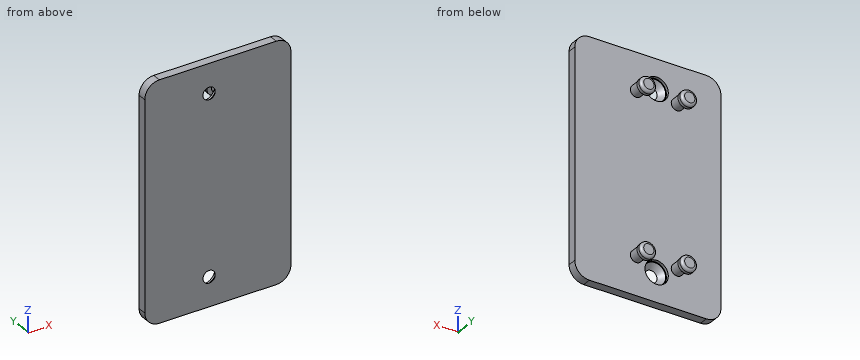
Autodesk Inventor part; units mm, degrees
ref_plane "YZ Plane" through (0, 0, 0) normal (1, 0, 0) x (0, 1, 0)
ref_plane "XZ Plane" through (0, 0, 0) normal (0, 1, 0) x (-1, 0, 0)
ref_plane "XY Plane" through (0, 0, 0) normal (0, 0, 1) x (1, 0, 0)
sketch "Esboço1" plane through (0, 0, 0) normal (0, 1, 0) x (-1, 0, 0)
  line L0 (-20, 37.5) -> (20, 37.5)
  line L1 (22, 35.5) -> (22, -35.5)
  line L2 (20, -37.5) -> (-20, -37.5)
  line L3 (-22, -35.5) -> (-22, 35.5)
  line L4 (-22, 37.5) -> (22, -37.5) construction
  line L5 (22, 37.5) -> (-22, -37.5) construction
  arc A0 (22, 35.5) -> (20, 37.5) centre (20, 35.5) ccw
  arc A1 (-20, 37.5) -> (-22, 35.5) centre (-20, 35.5) ccw
  arc A2 (-22, -35.5) -> (-20, -37.5) centre (-20, -35.5) ccw
  arc A3 (20, -37.5) -> (22, -35.5) centre (20, -35.5) ccw
  line L6 (-20, 40.5) -> (20, 40.5)
  line L7 (25, 35.5) -> (25, -35.5)
  line L8 (20, -40.5) -> (-20, -40.5)
  line L9 (-25, -35.5) -> (-25, 35.5)
  line L10 (-25, 40.5) -> (25, -40.5) construction
  line L11 (25, 40.5) -> (-25, -40.5) construction
  arc A4 (25, 35.5) -> (20, 40.5) centre (20, 35.5) ccw
  arc A5 (20, -40.5) -> (25, -35.5) centre (20, -35.5) ccw
  arc A6 (-25, -35.5) -> (-20, -40.5) centre (-20, -35.5) ccw
  arc A7 (-20, 40.5) -> (-25, 35.5) centre (-20, 35.5) ccw
  point P0 (0, 0)
  dimension "d0" = 75
  dimension "d1" = 44
  dimension "d2" = 2
  dimension "d3" = 3
  dimension "d4" = 3
  dimension "d5" = 5
extrude "Extrusão1" add sketch "Esboço1" along normal blind 3 contours L0 A0 L1 A3 L2 A2 L3 A1 | L6 A4 L7 A5 L8 A6 L9 A7
sketch "Esboço2" plane through (0, 3, 0) normal (0, 1, 0) x (1, 0, 0)
  circle A0 centre (-10, -27.5) radius 2
  circle A1 centre (-10, 27.5) radius 2
  circle A2 centre (4, -27.5) radius 2
  circle A3 centre (4, 27.5) radius 2
  line L0 (-20, -40.5) -> (20, -40.5)
  line L1 (20, 40.5) -> (-20, 40.5)
  point P0 (0, 0)
  dimension "d8" = 4
  dimension "d9" = 13
  dimension "d10" = 4
  dimension "d11" = 10
  dimension "d12" = 13
extrude "Extrusão2" add sketch "Esboço2" along normal blind 3.5
sketch "Esboço3" plane through (-10, 6.5, 27.5) normal (0, 1, 0) x (1, 0, 0)
  circle A0 centre (0, 0) radius 2
  circle A1 centre (14, 0) radius 2
  circle A2 centre (14, 55) radius 2
  circle A3 centre (0, 55) radius 2
  circle A4 centre (-0.75, 0) radius 2.75
  circle A5 centre (0, 0) radius 2
  circle A6 centre (13.25, 0) radius 2.75
  circle A7 centre (13.25, 55) radius 2.75
  circle A8 centre (-0.75, 55) radius 2.75
  circle A9 centre (0, 55) radius 2
  circle A10 centre (14, 55) radius 2
  point P0 (10, 27.5)
  dimension "d15" = 5.5
extrude "Extrusão3" add sketch "Esboço3" along normal blind 2 contours A0 | A4 | A1 | A6 | A2 | A7 | A3 | A8
fillet "Arredondamento1" radius 1 4 edges at (-13.5, 8.5, -27.5) (0.5, 8.5, -27.5) (-13.5, 8.5, 27.5) (0.5, 8.5, 27.5)
sketch "Esboço4" plane through (0, 3, 0) normal (0, 1, 0) x (1, 0, 0)
  circle A0 centre (-3, -30.5) radius 2.1
  circle A1 centre (-3, 30.5) radius 2.1
  line L0 (-20, -40.5) -> (20, -40.5)
  line L1 (20, 40.5) -> (-20, 40.5)
  line L2 (-25, 35.5) -> (-25, -35.5)
  circle A2 centre (-3, -30.5) radius 4
  circle A3 centre (-3, 30.5) radius 4
  point P0 (0, 0)
  dimension "d19" = 4.2
  dimension "d20" = 10
  dimension "d21" = 10
  dimension "d22" = 22
  dimension "d25" = 8
extrude "Extrusão4" cut sketch "Esboço4" against normal blind 10 contours A0 | A1
extrude "Extrusão5" cut sketch "Esboço4" against normal blind 1
sketch "Esboço5" plane through (-3, 2, 30.5) normal (0, 1, 0) x (1, 0, 0)
  circle A0 centre (0, 0) radius 3.75
  circle A1 centre (0, 0) radius 2.1
  circle A2 centre (0, 61) radius 4
  circle A3 centre (0, 61) radius 3.75
  point P0 (3, 30.5)
  dimension "d28" = 7.5
  dimension "d29" = 7.5
chamfer "Chanfro1" distance 2 distance2 1.65 1 edges at (-5.1, 2, 30.5) measured on face at (-0.9068, 0.6667, 30.669)
chamfer "Chanfro2" distance 2 distance2 1.65 1 edges at (-5.1, 2, -30.5) measured on face at (-0.9068, 0.6667, -30.331)
properties part number "SuportForWall"
Input: part model. Units: mm. Frame: model coordinates. Give positions to 0.01 mm unless a question says otherwise; leave off trailing zeros. Loops run counter-clockwise (first coordinate to the right, second up) from the corner with the lowest first, then second, coordinate; pieces in that order, holes last. Notation, with made-up numbers: (46, -25.75) -> (94, -25.75) arc R23 cw to (94, -1.75) -> close; hole circle Ø4 at (21, -18). An arc over 180 degrees is marked (long way). Use a Markdown table: item, result.
Q1. Section query C-C, the plane x = -15. Return the cut outline in (y, z), plus the area to 3 significant figures.
Entries:
| item | result |
|---|---|
| outline | (0, -40.5) -> (3, -40.5) -> (3, 40.5) -> (0, 40.5) -> close |
| area | 243 mm² |
Q2. Ray query, probe 1 along Z at (x, y) = (-3, 2.3); probe 2 along Z at (x, y) = (-3, 0.05); probe 3 along X at (y, z) = (2.75, -32). Return the intervals inside material, ascending. Write a range as from..to.
Entries:
| item | result |
|---|---|
| probe 1 | z = -40.5..-34.5, -26.5..26.5, 34.5..40.5 |
| probe 2 | z = -40.5..-32.64, -28.36..28.36, 32.64..40.5 |
| probe 3 | x = -25..-6.71, 0.71..25 |
Q3. Section query A-A, the plane y = 4.75. Return the cut outline in (x, z), plus the area to 3 significant figures.
Entries:
| item | result |
|---|---|
| outline | circle Ø4 at (-10, -27.5); circle Ø4 at (-10, 27.5); circle Ø4 at (4, -27.5); circle Ø4 at (4, 27.5) |
| area | 50.3 mm² |
Q4. Section query B-B, the plane z = -8. Return the cut outline in (x, y).
Entries:
| item | result |
|---|---|
| outline | (-25, 0) -> (25, 0) -> (25, 3) -> (-25, 3) -> close |
Q5. First-contact query: P1, Ø6.5, axis at x = -2.5, z = -31, coming from the +Y side; P2, Ø1.5, axis at x = -8, z = -11, coming from the +Y side; P3, Ø2, axis at y = 7.5, z = -28.5, coming from the +X side. Flat tips, straight axial feed; report the tip coordinate or a pass-through.
Entries:
| item | result |
|---|---|
| P1 | stops at y = 2 |
| P2 | stops at y = 3 |
| P3 | stops at x = 6 |
